from build123d import *

# Parameters (mm, degrees)
SKETCH1_R           = 10
BOSS_EXTRUDE1_DEPTH = 20
FILLET1_R           = 10
CUT_EXTRUDE1_REACH  = 106.881
SKETCH2_R           = 10
CUT_EXTRUDE2_REACH  = 106.881
SKETCH2_2_R         = 10
FILLET2_RADIUS      = 20
FILLET2_LENGTH      = 10
FILLET3_RADIUS      = 20
FILLET3_LENGTH      = 10


with BuildPart() as part:
    # Sketch1 → Boss-Extrude1 (new, symmetric)
    with BuildSketch(Plane.XY):
        with BuildLine():
            Line((0, 0), (0, 10))
            Line((0, 10), (-65, 10))
            ThreePointArc((-65, 10), (-90, -15), (-65, -40))
            Line((-65, -40), (0, -40))
            Line((0, -40), (0, -30))
            Line((0, -30), (-40, -30))
            Line((-40, -30), (-40, 0))
            Line((-40, 0), (0, 0))
        make_face()
        with Locations((-65, -15)):
            Circle(SKETCH1_R, mode=Mode.SUBTRACT)
    extrude(amount=BOSS_EXTRUDE1_DEPTH, both=True)

    # Fillet1
    fillet1_edges = [part.edges().sort_by_distance(p)[0] for p in [
        (-40, -15, -20),
        (-40, -15, 20),
    ]]
    fillet(fillet1_edges, radius=FILLET1_R)

    # Sketch2 → Cut-Extrude1 (cut, up to next)
    with BuildSketch(Plane(origin=(0, 10, 0), x_dir=(1, 0, 0), z_dir=(0, 1, 0)), mode=Mode.PRIVATE) as cut_extrude1_sk1:
        with Locations(Location((-20, 0, 0), (0, 0, 180))):
            Circle(SKETCH2_R)
    cut_extrude1_tool1 = extrude(cut_extrude1_sk1.sketch, amount=-CUT_EXTRUDE1_REACH, mode=Mode.PRIVATE) & part.part
    add(cut_extrude1_tool1.solids().sort_by_distance((-20, 10, 0))[0], mode=Mode.SUBTRACT)

    # Sketch2<2> → Cut-Extrude2 (cut, up to next)
    with BuildSketch(Plane(origin=(0, 10, 0), x_dir=(1, 0, 0), z_dir=(0, 1, 0)), mode=Mode.PRIVATE) as cut_extrude2_sk1:
        with Locations(Location((-20, 0, 0), (0, 0, 180))):
            Circle(SKETCH2_2_R)
    cut_extrude2_tool1 = extrude(cut_extrude2_sk1.sketch, amount=-CUT_EXTRUDE2_REACH, mode=Mode.PRIVATE) & part.part
    add(cut_extrude2_tool1.solids().sort_by_distance((-20, 10, 0))[0], mode=Mode.SUBTRACT)

    # Fillet2: full round fillet: the end face becomes a half cylinder, R = half its width
    fillet2_face = Plane((0, -35, 0), x_dir=(0, -1, 0), z_dir=(1, 0, 0))  # on the end face: x along it, z out of the body
    fillet2_slab = fillet2_face.offset(-FILLET2_RADIUS / 2) * Box(FILLET2_LENGTH, 2 * FILLET2_RADIUS, FILLET2_RADIUS, mode=Mode.PRIVATE)  # the body's end, R deep
    fillet2_round = Plane((-20, -35, 0), x_dir=(1, 0, 0), z_dir=(0, -1, 0)) * Cylinder(FILLET2_RADIUS, FILLET2_LENGTH, mode=Mode.PRIVATE)  # its axis R under the face
    add(fillet2_slab - fillet2_round, mode=Mode.SUBTRACT)

    # Fillet3: full round fillet: the end face becomes a half cylinder, R = half its width
    fillet3_face = Plane((0, 5, 0), x_dir=(0, 1, 0), z_dir=(1, 0, 0))  # on the end face: x along it, z out of the body
    fillet3_slab = fillet3_face.offset(-FILLET3_RADIUS / 2) * Box(FILLET3_LENGTH, 2 * FILLET3_RADIUS, FILLET3_RADIUS, mode=Mode.PRIVATE)  # the body's end, R deep
    fillet3_round = Plane((-20, 5, 0), x_dir=(1, 0, 0), z_dir=(0, 1, 0)) * Cylinder(FILLET3_RADIUS, FILLET3_LENGTH, mode=Mode.PRIVATE)  # its axis R under the face
    add(fillet3_slab - fillet3_round, mode=Mode.SUBTRACT)


solid = part.part
Work out the finished part from the listing and answer in its coordinate system (mm). A direction names the side the tool comes from. Give positions to 0.01 mm unless a question says otherwise; leave off trailing zeros. Order: outer loops, then holes, each group sorted by start corner. A loop starts at its lowest first (then second) coordinate and runs counter-clockwise, first axis right, second up. Notation, with made-up numbers: (69.25, 9) -> (108.25, 9) arc R20 ccw to (108.25, 46) -> close; hole circle Ø3 at (85.25, 17.25). An arc over 180 degrees is marked (long way). One line per item, written item: value.
Item 1: Find section D-D, the plane y = 1. Give the vertices of the cut face in (x, z).
Answer sheet:
outline: (-84.21, -20) -> (-20, -20) arc R20 ccw to (-20, 20) -> (-84.21, 20) -> close; hole circle Ø20 at (-20, 0)
Item 2: Find section C-C, the plane x = -44. Give the vertices of the cut face in (y, z), plus the area to 3 significant figures.
Answer sheet:
outline: (-40, -20) -> (-30, -20) -> (-30, -18) -> (0, -18) -> (0, -20) -> (10, -20) -> (10, 20) -> (0, 20) -> (0, 18) -> (-30, 18) -> (-30, 20) -> (-40, 20) -> close
area: 1,880 mm²
Item 3: Flat-ended cylindrical pins translate along their axes: P1, Ø5, axis at x = -16.5, y = -33.5, coming from the +Z side (3 decimals); P2, Ø1, axis at y = -15.5, z = -5, coming from the -X side; P3, Ø6, axis at y = -22, z = -4, coming from the +X side. Find the tip coordinate at first contact, or state that the pin passes through.
Answer sheet:
P1: z = 19.975
P2: x = -90
P3: x = -40
Item 4: Find section A-A, the plane z = 0. Give the vertices of the cut face in (x, y).
Answer sheet:
outline: (-65, -40) -> (-30, -40) -> (-30, -30) -> (-40, -30) -> (-40, 0) -> (-30, 0) -> (-30, 10) -> (-65, 10) arc R25 ccw to start; (-10, -40) -> (0, -40) -> (0, -30) -> (-10, -30) -> close; (-10, 0) -> (0, 0) -> (0, 10) -> (-10, 10) -> close; hole circle Ø20 at (-65, -15)
Item 5: Find section B-B, the plane y = -15. Give the vertices of the cut face in (x, z), plus the area to 3 significant figures.
Answer sheet:
outline: (-90, -20) -> (-75, -20) -> (-75, 20) -> (-90, 20) -> close; (-55, -20) -> (-50, -20) arc R10 ccw to (-40, -10) -> (-40, 10) arc R10 ccw to (-50, 20) -> (-55, 20) -> close
area: 1,160 mm²
Item 6: A tool of negligible diameter and unlimited length cuts with its end or side. For faces 1 (the flat face through (-55, -20, -20)), 2 (the cylindrical face through (-42.85, -14.79, 16.99)), 3 (the flat face through (-40, -15, 0)), from which of +Z, -Z, +X, -X, +Y, -Y can it reach the whole face along a straight path? Write none if from no direction.
Answer sheet:
face 1: -Z, +X, -X, +Y, -Y
face 2: +Z, +X
face 3: +Z, -Z, +X
Item 7: Determine the mould class of faces 4 (the cylindrical face through (-75, -15, 0)), 5 (the cylindrical face through (-89.994, -14.45, 0.28)), 6 (the flat face through (-30.2, -30, 0.3)), 7 (the cylindrical face through (-42.85, -14.79, -16.99)) for opening direction X: released by +X, released by -X, zero draft, split by the parting line, or undercut.
Answer sheet:
face 4: undercut
face 5: released by -X
face 6: zero draft
face 7: released by +X
Item 8: Straight lines are drawn through the part: probe 1 along Y at (x, z) = (-39.5, -3.5); probe 2 along Z at (x, y) = (-20, 4.25); probe 3 along Y at (x, z) = (-65, -5). For each, find the intervals that lie inside material, in ascending order.
Answer sheet:
probe 1: -40 to -30, 0 to 10
probe 2: -20 to -10, 10 to 20
probe 3: -40 to -25, -5 to 10
